Source: CAD feature listing. Evaluate the final solid. Frame: model axes, mm. Give positions to 0.01 mm unless a question says otherwise; leave off trailing zeros. Loops run counter-clockwise (first coordinate to the right, second up) from the corner with the lowest first, then second, coordinate; pieces in that order, holes last. Notation, with made-up numbers: (-22.5, 88) - (10.5, 88) arc R10 cw to (10.5, 105) - close; hole circle Ø4 at (12.5, 80.5). An arc over 180 degrees is marked (long way). Put each result on its own line as item: value.
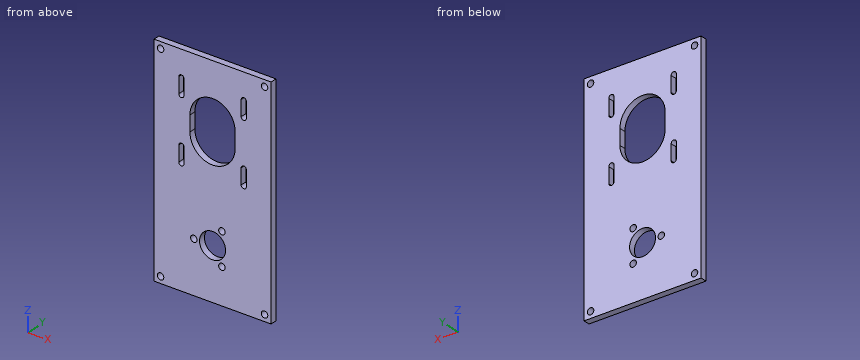
Autodesk Inventor part; units mm, degrees
ref_plane "YZ Plane" through (0, 0, 0) normal (1, 0, 0) x (0, 1, 0)
ref_plane "XZ Plane" through (0, 0, 0) normal (0, 1, 0) x (-1, 0, 0)
ref_plane "XY Plane" through (0, 0, 0) normal (0, 0, 1) x (1, 0, 0)
sketch "Sketch1" plane through (0, 0, 0) normal (0, 1, 0) x (-1, 0, 0)
  line L0 (0, 0) -> (57.15, 0)
  line L1 (57.15, 0) -> (57.15, -107.95)
  line L2 (57.15, -107.95) -> (0, -107.95)
  line L3 (0, -107.95) -> (0, 0)
  line L4 (57.15, -53.975) -> (0, -53.975) construction
  circle A0 centre (28.575, -35.56) radius 11.049
  line L5 (28.575, -35.56) -> (43.815, -35.56) construction
  line L6 (43.815, -35.56) -> (43.815, -50.8) construction
  line L7 (43.815, -50.8) -> (28.575, -50.8) construction
  line L8 (28.575, -50.8) -> (28.575, -35.56) construction
  line L9 (28.575, -35.56) -> (13.335, -35.56) construction
  line L10 (13.335, -35.56) -> (13.335, -20.32) construction
  line L11 (13.335, -20.32) -> (28.575, -20.32) construction
  line L12 (28.575, -20.32) -> (28.575, -35.56) construction
  line L13 (43.815, -50.8) -> (13.335, -50.8) construction
  line L14 (13.335, -50.8) -> (13.335, -20.32) construction
  line L15 (13.335, -20.32) -> (43.815, -20.32) construction
  line L16 (43.815, -20.32) -> (43.815, -50.8) construction
  circle A1 centre (43.815, -50.8) radius 1.27
  circle A2 centre (43.815, -20.32) radius 1.27
  circle A3 centre (13.335, -50.8) radius 1.27
  circle A4 centre (13.335, -20.32) radius 1.27
  line L17 (28.575, -107.95) -> (28.575, -53.975) construction
  line L18 (28.575, -35.56) -> (28.575, -27.94) construction
  circle A5 centre (28.575, -27.94) radius 11.049
  line L19 (43.815, -50.8) -> (43.815, -43.18) construction
  line L20 (13.335, -50.8) -> (13.335, -43.18) construction
  line L21 (13.335, -20.32) -> (13.335, -12.7) construction
  line L22 (43.815, -20.32) -> (43.815, -12.7) construction
  circle A6 centre (43.815, -43.18) radius 1.27
  circle A7 centre (13.335, -43.18) radius 1.27
  circle A8 centre (13.335, -12.7) radius 1.27
  circle A9 centre (43.815, -12.7) radius 1.27
  line L23 (45.085, -43.18) -> (45.085, -50.8)
  line L24 (42.545, -43.18) -> (42.545, -50.8)
  line L25 (14.605, -43.18) -> (14.605, -50.8)
  line L26 (12.065, -43.18) -> (12.065, -50.8)
  line L27 (12.065, -12.7) -> (12.065, -20.32)
  line L28 (14.605, -20.32) -> (14.605, -12.7)
  line L29 (45.085, -12.7) -> (45.085, -20.32)
  line L30 (42.545, -20.32) -> (42.545, -12.7)
  line L31 (28.575, -107.95) -> (28.575, -82.55) construction
  circle A10 centre (28.575, -82.55) radius 6.35
  line L32 (57.15, 0) -> (57.15, -12.7)
  line L33 (57.15, 0) -> (44.45, 0)
  line L34 (44.45, 0) -> (57.15, -12.7) construction
  line L35 (57.15, 0) -> (50.8, -6.35) construction
  line L36 (0, 0) -> (12.7, 0) construction
  line L37 (0, 0) -> (0, -12.7) construction
  line L38 (0, -12.7) -> (12.7, 0) construction
  line L39 (0, 0) -> (6.35, -6.35) construction
  line L40 (57.15, -107.95) -> (57.15, -95.25) construction
  line L41 (57.15, -107.95) -> (44.45, -107.95) construction
  line L42 (44.45, -107.95) -> (57.15, -95.25) construction
  line L43 (57.15, -107.95) -> (50.8, -101.6) construction
  line L44 (0, -107.95) -> (12.7, -107.95) construction
  line L45 (0, -107.95) -> (0, -95.25) construction
  line L46 (0, -95.25) -> (12.7, -107.95) construction
  line L47 (6.35, -101.6) -> (0, -107.95) construction
  circle A11 centre (53.975, -104.775) radius 1.5875
  circle A12 centre (3.175, -104.775) radius 1.5875
  circle A13 centre (53.975, -3.175) radius 1.5875
  circle A14 centre (3.175, -3.175) radius 1.5875
  line L48 (17.526, -35.56) -> (17.526, -27.94)
  line L49 (39.624, -35.56) -> (39.624, -27.94)
  line L50 (28.575, -82.55) -> (37.719, -82.55) construction
  line L51 (28.575, -82.55) -> (24.003, -74.6311) construction
  line L52 (28.575, -82.55) -> (24.003, -90.4689) construction
  circle A15 centre (24.003, -90.4689) radius 1.5875
  circle A16 centre (37.719, -82.55) radius 1.5875
  circle A17 centre (24.003, -74.6311) radius 1.5875
  point P0 (38.7216, -23.5665)
  point P1 (18.4284, -23.5665)
  dimension "d0" = 57.15
  dimension "d1" = 107.95
  dimension "d2" = 22.098
  dimension "d3" = 15.24
  dimension "d4" = 15.24
  dimension "d5" = 15.24
  dimension "d6" = 15.24
  dimension "d7" = 2.54
  dimension "d8" = 2.54
  dimension "d9" = 2.54
  dimension "d10" = 2.54
  dimension "d11" = 7.62
  dimension "d12" = 22.098
  dimension "d13" = 7.62
  dimension "d14" = 7.62
  dimension "d15" = 7.62
  dimension "d16" = 7.62
  dimension "d17" = 2.54
  dimension "d18" = 2.54
  dimension "d19" = 2.54
  dimension "d20" = 2.54
  dimension "d21" = 25.4
  dimension "d22" = 12.7
  dimension "d25" = 12.7
  dimension "d26" = 12.7
  dimension "d27" = 12.7
  dimension "d28" = 12.7
  dimension "d29" = 12.7
  dimension "d30" = 12.7
  dimension "d31" = 12.7
  dimension "d32" = 12.7
  dimension "d33" = 3.175
  dimension "d34" = 3.175
  dimension "d35" = 3.175
  dimension "d36" = 3.175
  dimension "d39" = 35.56
  dimension "d42" = 9.144
  dimension "d43" = 9.144
  dimension "d45" = 120
  dimension "d47" = 9.144
  dimension "d48" = 120
  dimension "d49" = 3.175
  dimension "d50" = 3.175
  dimension "d51" = 3.175
extrude "Extrusion4" add sketch "Sketch1" along normal blind 3.175
equation "\"d3\" = d5"
equation "\"d4\" = d6"
equation "\"d7\" = d10"
equation "\"d8\" = d10"
equation "\"d9\" = d10"
equation "\"d12\" = d2"
equation "\"d13\" = d11"
equation "\"d14\" = d11"
equation "\"d15\" = d11"
equation "\"d16\" = d11"
equation "\"d17\" = d10"
equation "\"d18\" = d10"
equation "\"d19\" = d10"
equation "\"d20\" = d10"
equation "\"d42\" = d47"
equation "\"d43\" = d47"
equation "\"d50\" = d49"
equation "\"d51\" = d49"
properties part number "lid"
1) Pin query (flat end, axial travel): P1, Ø12, axis at x = -29, z = -69, coming from the -Y side. Return the tip coordinate at first contact, or that it passes through.
Check result:
P1: y = 0
2) Section query D-D, the plane z = -48. Output: boundary loops of the cut face in (x, y) (3 decimals).
Check result:
outline: (-57.15, 0) - (-45.085, 0) - (-45.085, 3.175) - (-57.15, 3.175) - close; (-42.545, 0) - (-14.605, 0) - (-14.605, 3.175) - (-42.545, 3.175) - close; (-12.065, 0) - (0, 0) - (0, 3.175) - (-12.065, 3.175) - close
3) Material intervals for line 1 along X through (y, z) = (1.95, -12.5); line 2 along Z through (x, y) = (-3, 2.8); line 3 along X through (y, z) = (2.35, -16) (3 decimals), sorted ascending. Write a range as [from, to].
Check result:
line 1: [-57.15, -45.07], [-42.56, -14.59], [-12.08, 0]
line 2: [-107.95, -106.35], [-103.2, -4.75], [-1.6, 0]
line 3: [-57.15, -45.085], [-42.545, -14.605], [-12.065, 0]
4) Section query B-B, the plane z = -34. Output: boundary loops of the cut face in (x, y) (3 decimals).
Check result:
outline: (-57.15, 0) - (-39.624, 0) - (-39.624, 3.175) - (-57.15, 3.175) - close; (-17.526, 0) - (0, 0) - (0, 3.175) - (-17.526, 3.175) - close
5) Section query A-A, the plane z = -82.55. State how many separate pieces and enclosed holes the cut face has, plus the area to 3 significant figures.
Check result:
separate pieces: 3
enclosed holes: 0
area: 131 mm²
